from build123d import *

# Parameters (mm, degrees)
F0_R     = 4
F1_DEPTH = 6
F2_W     = 8
F2_H     = 8
F3_DEPTH = 15
F4_R     = 4
F5_DEPTH = 6


with BuildPart() as f1:
    # F0 (on Top) → F1 (new body)
    with BuildSketch(Plane.XY):
        Circle(F0_R)
    extrude(amount=F1_DEPTH)

    # F2 (on face) → F3 (join)
    with BuildSketch(Plane.XY.offset(6)):
        Rectangle(F2_W, F2_H)
    extrude(amount=F3_DEPTH)

    # F4 (on face) → F5 (join)
    with BuildSketch(Plane.XY.offset(21)):
        Circle(F4_R)
    extrude(amount=F5_DEPTH)


solid = f1.part
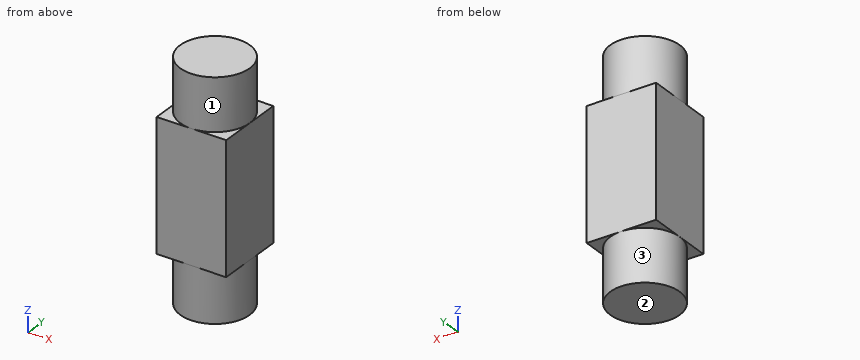
Verification items for the finished model (mm, model axes). Face numbers are marked on the shaded views. A direction names the side the tool comes from. Coordinates: 2 decimals unless noted, no trailing zeros. Write each loop counter-clockwise with the first axis right and the second up, starting at its lowest first coordinate (ties: lowest second). Pieces come first, ordered by that corner, then holes. Notation, with made-up numbers: (50, 82.5) - (96, 82.5) arc R21 cw to (96, 119.5) - close; hole circle Ø4 at (81.25, -0.5). An arc over 180 degrees is marked (long way). Answer as a JSON object with one key per item and string values.
(1) Cross-section at A-A on z = 5.25. Record the cut outline in (x, y).
Report:
{"outline": "circle Ø8 at (0, 0)"}
(2) Cross-section at B-B on y = 3.25. Record the cut outline in (x, z).
Report:
{"outline": "(-4, 6) - (-2.33, 6) - (-2.33, 0) - (2.33, 0) - (2.33, 6) - (4, 6) - (4, 21) - (2.33, 21) - (2.33, 27) - (-2.33, 27) - (-2.33, 21) - (-4, 21) - close"}
(3) Cross-section at C-C on x = 3. Record the cut outline in (y, z), plus the area to 3 significant figures.
Report:
{"outline": "(-4, 6) - (-2.65, 6) - (-2.65, 0) - (2.65, 0) - (2.65, 6) - (4, 6) - (4, 21) - (2.65, 21) - (2.65, 27) - (-2.65, 27) - (-2.65, 21) - (-4, 21) - close", "area": "183 mm^2"}
(4) Tool access check on the marked faces 1, 2 and 3. Record the directions out of +Z, -Z, +X, -X, +Y, -Y that give a thin tool (end or side, any length) a straight path to the whole face; none if there is none.
Report:
{"face 1": "+Z", "face 2": "-Z, +X, -X, +Y, -Y", "face 3": "-Z"}
(5) Thickness scan on line 1 along Z through (x, y) = (3.5, 3.25); line 2 along X through (y, z) = (0.75, 24.5); line 3 along Y through (x, z) = (-2.5, 23). Record the ranges inside material, lowest first.
Report:
{"line 1": "6 to 21", "line 2": "-3.93 to 3.93", "line 3": "-3.12 to 3.12"}
